Source: CAD feature listing. Evaluate the final solid. Frame: model axes, mm. A direction names the side the tool comes from. Round coordinates to 2 decimals unless told otherwise and drop trailing zeros. Write each loop counter-clockwise with the first axis right and the second up, starting at its lowest first coordinate (ties: lowest second). Pieces come first, ordered by that corner, then holes. Notation, with made-up numbers: M -29,86 L -3,86 A19 cw -3,100 Z; hole C 82.25,84 d10. An arc over 180 degrees is marked long. Answer in a Markdown table with one row per item.
from build123d import *

# Parameters (mm, degrees)
SKETCH1_W                                       = 10
SKETCH1_H                                       = 262
BOSS_EXTRUDE1_DEPTH                             = 42
CBORE_FOR_M5_SOCKET_HEAD_CAP_SCREW1_D           = 5.5
CBORE_FOR_M5_SOCKET_HEAD_CAP_SCREW1_CBORE_D     = 10
CBORE_FOR_M5_SOCKET_HEAD_CAP_SCREW1_CBORE_DEPTH = 5
CBORE_FOR_M5_SOCKET_HEAD_CAP_SCREW2_D           = 5.5
CBORE_FOR_M5_SOCKET_HEAD_CAP_SCREW2_CBORE_D     = 10
CBORE_FOR_M5_SOCKET_HEAD_CAP_SCREW2_CBORE_DEPTH = 5
CHAMFER1_SIZE                                   = 50


with BuildPart() as part:
    # Sketch1 → Boss-Extrude1 (new, symmetric)
    with BuildSketch(Plane(origin=(0, 0, 0), x_dir=(0, 0, -1), z_dir=(1, 0, 0))):
        with Locations((-5, 131)):
            Rectangle(SKETCH1_W, SKETCH1_H)
    extrude(amount=BOSS_EXTRUDE1_DEPTH, both=True)

    # CBORE for M5 Socket Head Cap Screw1 (through all)
    with Locations(Plane(origin=(0, 0, 0), x_dir=(-1, 0, 0), z_dir=(0, 0, -1))):
        with Locations((36, 256), (36, 212), (36, 168)):
            CounterBoreHole(CBORE_FOR_M5_SOCKET_HEAD_CAP_SCREW1_D / 2, CBORE_FOR_M5_SOCKET_HEAD_CAP_SCREW1_CBORE_D / 2, CBORE_FOR_M5_SOCKET_HEAD_CAP_SCREW1_CBORE_DEPTH)

    # CBORE for M5 Socket Head Cap Screw2 (through all)
    with Locations(Plane(origin=(0, 0, 0), x_dir=(-1, 0, 0), z_dir=(0, 0, -1))):
        with Locations((-25, 6), (25, 6)):
            CounterBoreHole(CBORE_FOR_M5_SOCKET_HEAD_CAP_SCREW2_D / 2, CBORE_FOR_M5_SOCKET_HEAD_CAP_SCREW2_CBORE_D / 2, CBORE_FOR_M5_SOCKET_HEAD_CAP_SCREW2_CBORE_DEPTH)

    # Chamfer1
    chamfer1_edges = [part.edges().sort_by_distance(p)[0] for p in [
        (42, 262, 5),
    ]]
    chamfer(chamfer1_edges, length=CHAMFER1_SIZE)


solid = part.part
Q1. Section D-D (z = 7.5). Return loops of the section in (x, y), and give its area (3 significant figures).
Solutions:
| item | result |
|---|---|
| outline | M -42,0 L 42,0 L 42,212 L -8,262 L -42,262 Z; hole C -36,168 d5.5; hole C -36,212 d5.5; hole C -36,256 d5.5; hole C -25,6 d5.5; hole C 25,6 d5.5 |
| area | 20,600 mm2 |
Q2. Section C-C (y = 256). Return loops of the section in (x, z).
Solutions:
| item | result |
|---|---|
| outline | M -42,0 L -41,0 L -41,5 L -38.75,5 L -38.75,10 L -42,10 Z; M -33.25,5 L -31,5 L -31,0 L -2,0 L -2,10 L -33.25,10 Z |
Q3. Section A-A (x = -25). Return loops of the section in (y, z).
Solutions:
| item | result |
|---|---|
| outline | M 0,0 L 1,0 L 1,5 L 3.25,5 L 3.25,10 L 0,10 Z; M 8.75,5 L 11,5 L 11,0 L 262,0 L 262,10 L 8.75,10 Z |
Q4. Access query for faces 4 (the flat face through (-38.2, 209.8, 5)), 5 (the flat face through (1, 129, 0)). Directions: +Z, -Z, +X, -X, +Y, -Y. A direction counts if a zero-diameter tool reaches every point of the face in a straight line with its end or side. Return the directions, or none.
Solutions:
| item | result |
|---|---|
| face 4 | -Z |
| face 5 | -Z, +X, -X, +Y, -Y |
Q5. Section B-B (x = -36). Return loops of the section in (y, z), and give its area (3 significant figures).
Solutions:
| item | result |
|---|---|
| outline | M 0,0 L 163,0 L 163,5 L 165.25,5 L 165.25,10 L 0,10 Z; M 170.75,5 L 173,5 L 173,0 L 207,0 L 207,5 L 209.25,5 L 209.25,10 L 170.75,10 Z; M 214.75,5 L 217,5 L 217,0 L 251,0 L 251,5 L 253.25,5 L 253.25,10 L 214.75,10 Z; M 258.75,5 L 261,5 L 261,0 L 262,0 L 262,10 L 258.75,10 Z |
| area | 2,390 mm2 |
Q6. Pull-direction query (X, two-part tool) for faces 1 (the flat face through (-25, 262, 5)), 2 (the flat face through (17, 237, 5)), 3 (the cylindrical face through (-27.747, 6.121, 7.535)); classes: pulls with the +X half, pulls with the -X half, needs draft (parallel to the pull), parting line crosses it, or undercut.
Solutions:
| item | result |
|---|---|
| face 1 | needs draft |
| face 2 | pulls with the +X half |
| face 3 | undercut |
Q7. Contact query for flat-ended pins moving along their axis: pin 1 Ø3 at (x, z) = (17.5, 8) entering from +Y; pin 2 Ø5 at (x, y) = (15, 77) entering from -Z; pin 3 Ø6.5 at (x, y) = (-36, 168) entering from -Z. Output: stop coordinate, or through.
Solutions:
| item | result |
|---|---|
| pin 1 | stops at y = 238 |
| pin 2 | stops at z = 0 |
| pin 3 | stops at z = 5 |
Q8. Material intervals for probe 1 along Y at (x, z) = (-36, 7.5); probe 2 along Y at (x, z) = (-36, 3.65); probe 3 along Y at (x, z) = (-25, 8.1), sorted ascending.
Solutions:
| item | result |
|---|---|
| probe 1 | y = 0 to 165.25, 170.75 to 209.25, 214.75 to 253.25, 258.75 to 262 |
| probe 2 | y = 0 to 163, 173 to 207, 217 to 251, 261 to 262 |
| probe 3 | y = 0 to 3.25, 8.75 to 262 |
